Can you work these out from the drawing? Everything is in mm from the part's minimum corner. A direction names the side the tool comes from. Round coordinates to 2 decimals unless told otherwise and drop trailing zeros. Loops run counter-clockwise (first coordinate to the right, second up) from the corner with the lowest first, then second, coordinate; pieces in that order, holes last. Notation, with made-up numbers: (65.25, 23.25) - (90.25, 23.25) arc R22 ccw to (90.25, 44.25) - close; hole circle Ø10 at (68.5, 35.5). An arc over 180 degrees is marked (long way). Answer as CSV lines item,"result". Start each with the question number.
1) Suppose I cut it at D-D, the plane x = 48. Write out the boundary of the cut face in (y, z).
2) Which directions (+Z, -Z, +X, -X, +Y, -Y) give clear straight access to the entire face, cutting with the end or side of a thin tool? Please do the marked faces 1 and 2.
3) I'm going to push flat-ended pins straight in: pin 1 Ø4 at (x, y) = (59.5, 8) entering from -Z; pin 2 Ø12 at (x, z) = (61, 77) entering from +Y; pin 3 Ø1.5 at (x, y) = (22, 16.5) entering from +Z. Where does each tip first touch, or does it pass through?
4) We'd pull the mould along Y, two halves only. Please class the marked faces 3, 4 and 5: pulls with the +Y half, pulls with the -Y half, needs draft (parallel to the pull), parting line crosses it, or undercut.
5) Suppose I cut it at A-A, the plane x = 66.5. Write out the boundary of the cut face in (y, z).
6) Please list where these lines run through material, in increasing order: line 1 along X through (y, z) = (10.75, 114) (1 decimal); line 2 along Z through (x, y) = (44.5, 23.5); line 3 along X through (y, z) = (14, 108) (1 decimal).
7) Suppose I cut it at B-B, the plane z = 54. Write out the boundary of the cut face in (x, y).
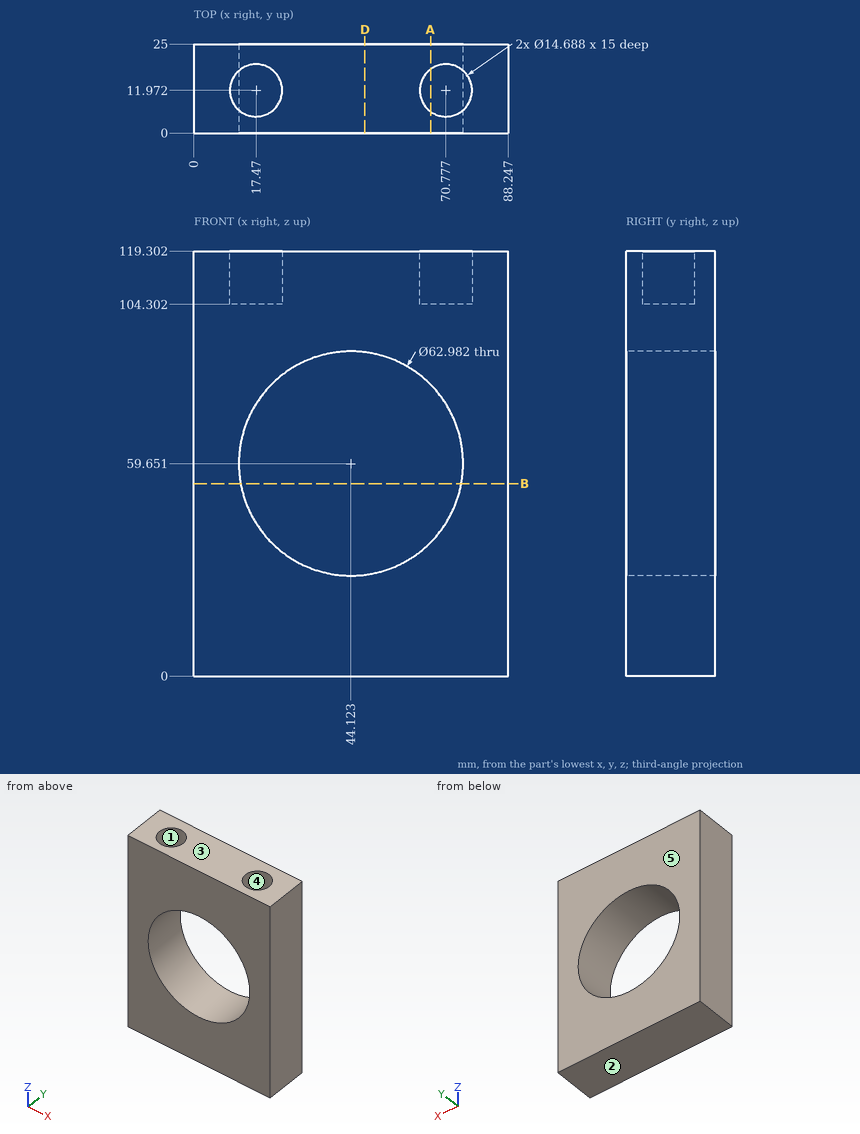
Filled sheet:
1,outline,"(0, 0) - (25, 0) - (25, 28.4) - (0, 28.4) - close; (0, 90.9) - (25, 90.9) - (25, 119.3) - (0, 119.3) - close"
2,face 1,"+Z"
2,face 2,"-Z, +X, -X, +Y, -Y"
3,pin 1,"z = 0"
3,pin 2,"through"
3,pin 3,"z = 104.3"
4,face 3,"needs draft"
4,face 4,"undercut"
4,face 5,"pulls with the +Y half"
5,outline,"(0, 0) - (25, 0) - (25, 37.49) - (0, 37.49) - close; (0, 81.81) - (25, 81.81) - (25, 119.3) - (17.94, 119.3) - (17.94, 104.3) - (6, 104.3) - (6, 119.3) - (0, 119.3) - close"
6,line 1,"0 to 10.2, 24.7 to 63.5, 78 to 88.2"
6,line 2,"0 to 28.16, 91.14 to 119.3"
6,line 3,"0 to 10.4, 24.5 to 63.7, 77.8 to 88.2"
7,outline,"(0, 0) - (13.14, 0) - (13.14, 25) - (0, 25) - close; (75.1, 0) - (88.25, 0) - (88.25, 25) - (75.1, 25) - close"
